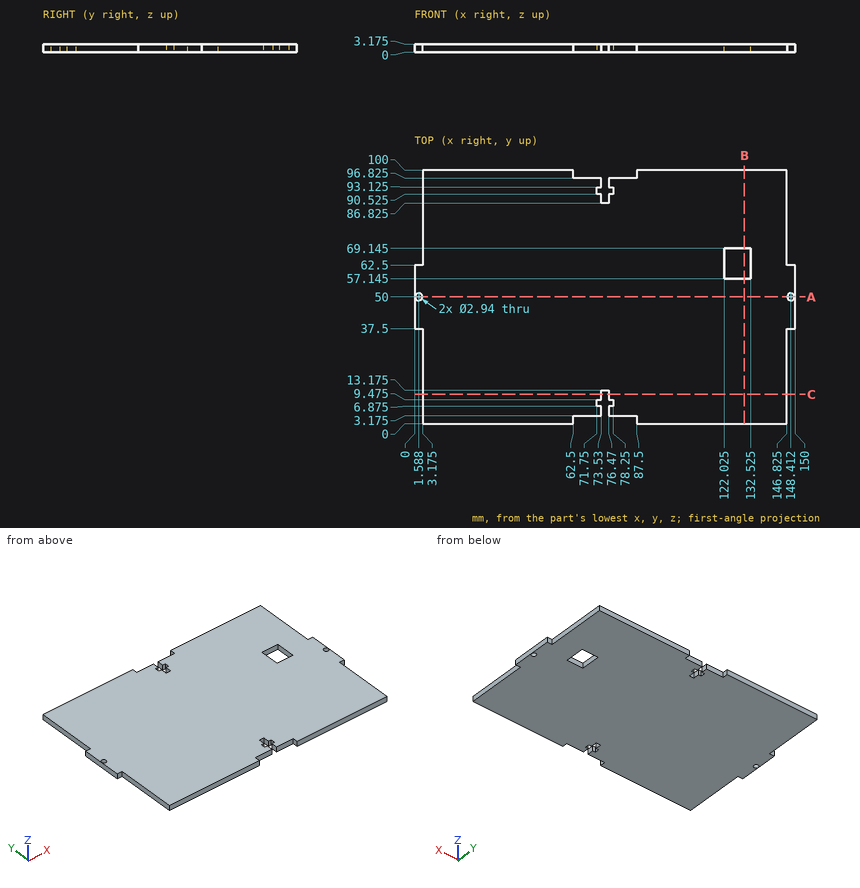
Could you check a few things on this drawing? It's one solid part, dimensions in mm from its lowest x, y, z. Round coordinates to 2 decimals unless told otherwise and drop trailing zeros. Order: outer loops, then holes, each group sorted by start corner. A loop starts at its lowest first (then second) coordinate and runs counter-clockwise, first axis right, second up.
(1) Imagine slicing it at B-B (x = 130). Write out the boundary of the cut face in (y, z) (1 decimal).
Response values:
outline: (0, 0) - (57.1, 0) - (57.1, 3.2) - (0, 3.2) - close; (69.1, 0) - (100, 0) - (100, 3.2) - (69.1, 3.2) - close
(2) I'm going to push flat-ended pins straight in: pin 1 (0.5 mm diameter, centred on x = 72.5, z = 1.5, fed in from +Y) (1 decimal); pin 2 (1 mm diameter, centred on x = 95.5, z = 2.5, fed in from -Y); pin 3 (0.8 mm diameter, centred on y = 8, z = 2, fed in from -X) (1 decimal); pin 4 (0.8 mm diameter, centred on y = 91.5, z = 2, fed in from +X) (1 decimal). Where does each tip first touch, or does it pass through?
Response values:
pin 1: stops at y = 96.8
pin 2: stops at y = 0
pin 3: stops at x = 3.2
pin 4: stops at x = 146.8
(3) Imagine slicing it at A-A (y = 50). Count the separate pieces of the cut face and the enclosed holes in it.
Response values:
separate pieces: 3
enclosed holes: 0
(4) Please list where these lines run through material, in increasing order: line 1 along X through (y, z) = (69, 1.15) (1 decimal); line 2 along X through (y, z) = (49, 1.85) (1 decimal); line 3 along X through (y, z) = (11.5, 2.95) (1 decimal).
Response values:
line 1: x = 3.2 to 122, 132.5 to 146.8
line 2: x = 0 to 0.5, 2.7 to 147.3, 149.5 to 150
line 3: x = 3.2 to 73.5, 76.5 to 146.8
(5) Imagine slicing it at C-C (y = 11.5). Write out the boundary of the cut face in (x, z) (1 decimal).
Response values:
outline: (3.2, 0) - (73.5, 0) - (73.5, 3.2) - (3.2, 3.2) - close; (76.5, 0) - (146.8, 0) - (146.8, 3.2) - (76.5, 3.2) - close
